Can you work these out from the model? Positions are in its coordinate system, mm. Face numbers are marked on the shaded views. Give positions to 0.01 mm unless a question says otherwise; leave off trailing zeros. Write each loop counter-clockwise with the first axis right and the second up, starting at its lowest first coordinate (ties: lowest second). Pieces come first, ordered by that corner, then holes.
Autodesk Inventor part; units mm, degrees
ref_plane "YZ Plane" through (0, 0, 0) normal (1, 0, 0) x (0, 1, 0)
ref_plane "XZ Plane" through (0, 0, 0) normal (0, 1, 0) x (-1, 0, 0)
ref_plane "XY Plane" through (0, 0, 0) normal (0, 0, 1) x (1, 0, 0)
sketch "Sketch1" plane through (0, 0, 0) normal (0, 0, 1) x (1, 0, 0)
  circle A0 centre (0, 0) radius 4
  dimension "d0" = 8
extrude "Extrusion1" add sketch "Sketch1" along normal mid plane 59.0042
sketch "Sketch2" plane through (0, 0, 29.5021) normal (0, 0, 1) x (1, 0, 0)
  circle A0 centre (0, 0) radius 4 construction
  circle A1 centre (0, 0) radius 4 construction
  line L0 (-2.6458, 3) -> (2.6458, 3)
  line L1 (2.6458, -3) -> (-2.6458, -3)
  line L2 (0, 3) -> (0, -3) construction
  arc A2 (2.6458, 3) -> (-2.6458, 3) centre (0, 0) ccw
  arc A3 (-2.6458, -3) -> (2.6458, -3) centre (0, 0) ccw
  dimension "d3" = 6
extrude "Extrusion2" cut sketch "Sketch2" against normal blind 7.0104
sketch "Sketch3" plane through (-2.6458, 3, 29.5021) normal (0, 1, 0) x (1, 0, 0)
  line L0 (5.2915, 7.0104) -> (0, 7.0104) construction
  point P0 (2.6458, 29.5021)
  point P1 (2.6458, 4.0104)
  point P2 (2.6458, 7.0104)
  dimension "d6" = 3
hole "Hole1" at (0, 3, 25.4917) direction (0, -1, 0) diameter 4.4958 end through all
properties part number "rod" material "Aluminum 6061"
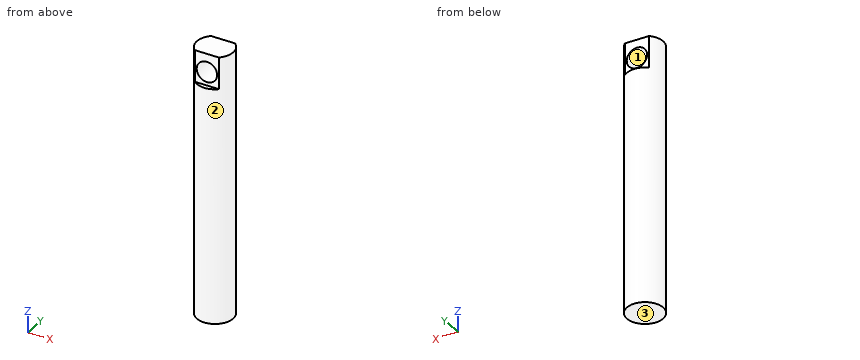
1) Suppose I cut it at D-D on y = -3.5. Write out the boundary of the cut face in (x, z).
Values follow:
outline: (-1.94, -29.5) - (1.94, -29.5) - (1.94, 22.49) - (-1.94, 22.49) - close
2) If we mould it in two halves opening along X, with no side actions, what happens to the marked faces 1, 2 and 3? For each: +X half, -X half, draft (parallel to the pull), parting line (faces both ways), or undercut.
Values follow:
face 1: undercut
face 2: parting line
face 3: draft
3) Suppose I cut it at A-A on x = 0. Write out the boundary of the cut face in (y, z).
Values follow:
outline: (-4, -29.5) - (4, -29.5) - (4, 22.49) - (3, 22.49) - (3, 23.24) - (-3, 23.24) - (-3, 22.49) - (-4, 22.49) - close; (-3, 27.74) - (3, 27.74) - (3, 29.5) - (-3, 29.5) - close
4) Please list where these lines run through material, in increasing order: L1, parallel to Z at x = 0, y = 0.5; L2, parallel to Z at x = -0.25, y = 3.5; L3, parallel to X at y = -0.25, z = -12.5.
Values follow:
L1: z = -29.5 to 23.24, 27.74 to 29.5
L2: z = -29.5 to 22.49
L3: x = -3.99 to 3.99
5) Suppose I cut it at B-B on y = 0. Write out the boundary of the cut face in (x, z), plus the area to 3 significant figures.
Values follow:
outline: (-4, -29.5) - (4, -29.5) - (4, 29.5) - (-4, 29.5) - close; hole circle Ø4.5 at (0, 25.49)
area: 456 mm2
6) For pin 1 Ø3.5 at (x, z) = (0, 25.49) entering from +Y; pin 2 Ø0.8 at (x, y) = (1, -3.5) entering from +Z; pin 3 Ø2.5 at (x, z) = (-0.5, 24.5) entering from -Y; pin 4 Ø1 at (y, z) = (-3, 5.5) entering from -X, each with a flat end and sliding along its axis, tell me the tip position at first contact or that it passes through.
Values follow:
pin 1: passes through
pin 2: stops at z = 22.49
pin 3: stops at y = -3
pin 4: stops at x = -3.12
7) Suppose I cut it at C-C on z = -15.5. Write out the boundary of the cut face in (x, y), plus the area to 3 significant figures.
Values follow:
outline: circle Ø8 at (0, 0)
area: 50.3 mm2
